```python
from build123d import *

# Parameters (mm, degrees)
SKETCH1_W           = 45.36
SKETCH1_H           = 20
BOSS_EXTRUDE1_DEPTH = 3.33
SKETCH2_R           = 8
SKETCH2_R_2         = 7.201770051
BOSS_EXTRUDE2_DEPTH = 11.5
SKETCH3_R           = 0.77
CUT_EXTRUDE1_DEPTH  = 11.5
SKETCH4_W           = 11
SKETCH4_H           = 4.71
BOSS_EXTRUDE3_DEPTH = 3
SKETCH5_W           = 10.29
SKETCH5_H           = 8.7
BOSS_EXTRUDE4_DEPTH = 3


with BuildPart() as part:
    # Sketch1 → Boss-Extrude1 (new body)
    with BuildSketch(Plane(origin=(0, 0, 0), x_dir=(1, 0, 0), z_dir=(0, 1, 0))):
        Rectangle(SKETCH1_W, SKETCH1_H)
    extrude(amount=BOSS_EXTRUDE1_DEPTH)

    # Sketch2 → Boss-Extrude2 (add)
    with BuildSketch(Plane(origin=(0, 3.33, 0), x_dir=(1, 0, 0), z_dir=(0, 1, 0))):
        with Locations(Location((12.68, 0, 0), (0, 0, 90))):
            Circle(SKETCH2_R)
        with Locations(Location((-12.68, 0, 0), (0, 0, 90))):
            Circle(SKETCH2_R_2)
    extrude(amount=BOSS_EXTRUDE2_DEPTH)

    # Sketch3 → Cut-Extrude1 (cut)
    with BuildSketch(Plane(origin=(0, 3.33, 0), x_dir=(1, 0, 0), z_dir=(0, 1, 0))):
        with Locations(Location((21.68, 9, 0), (0, 0, 270))):
            Circle(SKETCH3_R)
        with Locations(Location((21.68, -9, 0), (0, 0, 270))):
            Circle(SKETCH3_R)
        with Locations(Location((-21.68, -9, 0), (0, 0, 270))):
            Circle(SKETCH3_R)
        with Locations(Location((-21.68, 9, 0), (0, 0, 270))):
            Circle(SKETCH3_R)
    extrude(amount=-CUT_EXTRUDE1_DEPTH, mode=Mode.SUBTRACT)

    # Sketch4 → Boss-Extrude3 (add)
    with BuildSketch(Plane(origin=(0, 3.33, 0), x_dir=(1, 0, 0), z_dir=(0, 1, 0))):
        with Locations((0, 7.63)):
            Rectangle(SKETCH4_W, SKETCH4_H)
    extrude(amount=BOSS_EXTRUDE3_DEPTH)

    # Sketch5 → Boss-Extrude4 (add)
    with BuildSketch(Plane.XZ):
        with Locations((-1.239937646, 11.81)):
            Rectangle(SKETCH5_W, SKETCH5_H)
    extrude(amount=BOSS_EXTRUDE4_DEPTH)


solid = part.part
```
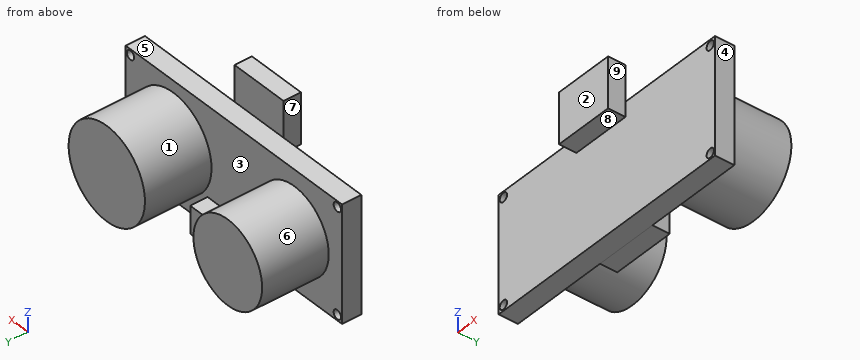
Work out the finished part from the listing and answer in its coordinate system (mm). Face numbers are marked on the shaded views. A direction names the side the tool comes from. Coordinates: 2 decimals unless noted, no trailing zeros. Write each loop counter-clockwise with the first axis right and the second up, starting at its lowest first coordinate (ties: lowest second). Pieces come first, ordered by that corner, then holes.
Q1. A cutting plane is placed at C-C, the plane y = 5.25. Give the vertices of the cut face in (x, z) (3 decimals).
Q2. Find the intervals of material crossed by line 1 (X direction, y = 2.5, z = -9); line 2 (Z direction, x = 17.5, y = 3.25); line 3 (Y direction, x = 18, z = 4.5), in increasing order.
Q3. Determine the mould class of the marked faces 1, 2, 3 and 4 for opening direction X: released by +X, released by -X, zero draft, split by the parting line, or undercut.
Q4. Which of the six approach directions +Z, -Z, +X, -X, +Y, -Y give full straight-line access (tool end or side, diameter ignored) to the marked faces 5, 6, 7, 8 and 9?
Q5. A cutting plane is placed at B-B, the plane z = -9. Give the vertices of the cut face in (x, y), then the cut area to 3 significant figures.
Q6. Each of these flat-tipped pins is pushed along its axis until it touches: pin 1 Ø1 at (x, z) = (-9, 8) entering from +Y; pin 2 Ø2 at (x, z) = (-21.68, -9) entering from -Y; pin 3 Ø0.9 at (x, y) = (-1.5, 5) entering from -Z (3 decimals). Where does it stop, or does it pass through?
Q7. A cutting plane is placed at D-D, the plane y = 2.5. Give the vertices of the cut face in (x, z), then the cut area to 3 significant figures.
Q8. A cutting plane is placed at A-A, the plane x = 21.68. Give the vertices of the cut face in (y, z), then the cut area to 3 significant figures.
Findings below:
1. outline: circle Ø14.404 at (-12.68, 0); (-5.5, -9.985) - (5.5, -9.985) - (5.5, -5.275) - (-5.5, -5.275) - close; circle Ø16 at (12.68, 0)
2. line 1: x = -22.68 to -22.45, -20.91 to 20.91, 22.45 to 22.68
2. line 2: z = -10 to 10
2. line 3: y = 0 to 14.83
3. face 1: undercut
3. face 2: zero draft
3. face 3: undercut
3. face 4: released by +X
4. face 5: +Z, +X, -X, +Y
4. face 6: +Y
4. face 7: +Z, -Z, -X, -Y
4. face 8: -Z, +X, -X, -Y
4. face 9: +Z, -Z, +X, -Y
5. outline: (-22.68, 0) - (-22.45, 0) - (-22.45, 3.33) - (-22.68, 3.33) - close; (-20.91, 0) - (20.91, 0) - (20.91, 3.33) - (5.5, 3.33) - (5.5, 6.33) - (-5.5, 6.33) - (-5.5, 3.33) - (-20.91, 3.33) - close; (22.45, 0) - (22.68, 0) - (22.68, 3.33) - (22.45, 3.33) - close
5. area: 174 mm2
6. pin 1: stops at y = 3.33
6. pin 2: stops at y = 0
6. pin 3: stops at z = -9.985
7. outline: (-22.68, -10) - (22.68, -10) - (22.68, 10) - (-22.68, 10) - close; hole circle Ø1.54 at (-21.68, -9); hole circle Ø1.54 at (-21.68, 9); hole circle Ø1.54 at (21.68, -9); hole circle Ø1.54 at (21.68, 9)
7. area: 900 mm2
8. outline: (0, -10) - (3.33, -10) - (3.33, -9.77) - (0, -9.77) - close; (0, -8.23) - (3.33, -8.23) - (3.33, 8.23) - (0, 8.23) - close; (0, 9.77) - (3.33, 9.77) - (3.33, 10) - (0, 10) - close
8. area: 56.3 mm2
